The figure shows three views and two pictorial views of one solid part (mm, origin at its lowest corner). Answer the questions. A direction names the side the tool comes from. Give positions to 0.01 mm unless a question says otherwise; leave off trailing zeros. Order: outer loops, then holes, each group sorted by start corner. A loop starts at its lowest first (then second) coordinate and runs counter-clockwise, first axis right, second up. Notation, with made-up numbers: (-3, 22) - (42, 22) arc R16 cw to (42, 30) - close; hole circle Ø1 at (4, 43). An arc over 180 degrees is marked (long way). Answer as a JSON object with one key per item and string values. Group by question number.
Q1. The mould has two halves that part along X. Classify the marked faces 1, 2 and 3: released by +X, released by -X, zero draft, split by the parting line, or undercut.
Q2. Given pin 1 (4 mm diameter, centred on x = 20, y = 5, fed in from -Z); pin 2 (8 mm diameter, centred on x = 33.44, y = 10.56, fed in from -Z); pin 3 (4 mm diameter, centred on x = 26.5, z = 26.5, fed in from -Y); pin 4 (8 mm diameter, centred on x = 25.5, z = 9, fed in from -Y), each flat-ended and moving along its own axis, determine where each tip first touches the part or whether it passes through.
Q3. Consider line 1 (Y direction, x = 20, z = 23); line 2 (Z direction, x = 23, y = 45.5); line 3 (Y direction, x = 26, z = 31). Determine where each line is inside the solid, lowest interval first.
Q4. For the marked faces 4 and 5, determine the directions among +Z, -Z, +X, -X, +Y, -Y from which every point of the face is accessible in a straight line to the end or side of a thin tool.
Q5. A cutting plane is placed at B-B, the plane x = 20. Give the vertices of the cut face in (y, z), and give its area (3 significant figures).
Q6. A cutting plane is placed at C-C, the plane x = 33. Give the vertices of the cut face in (y, z), and give its area (3 significant figures).
Q7. A cutting plane is placed at D-D, the plane x = 15. Give the vertices of the cut face in (y, z) (3 decimals).
Q8. A cutting plane is placed at A-A, the plane y = 24. Give the vertices of the cut face in (x, z).
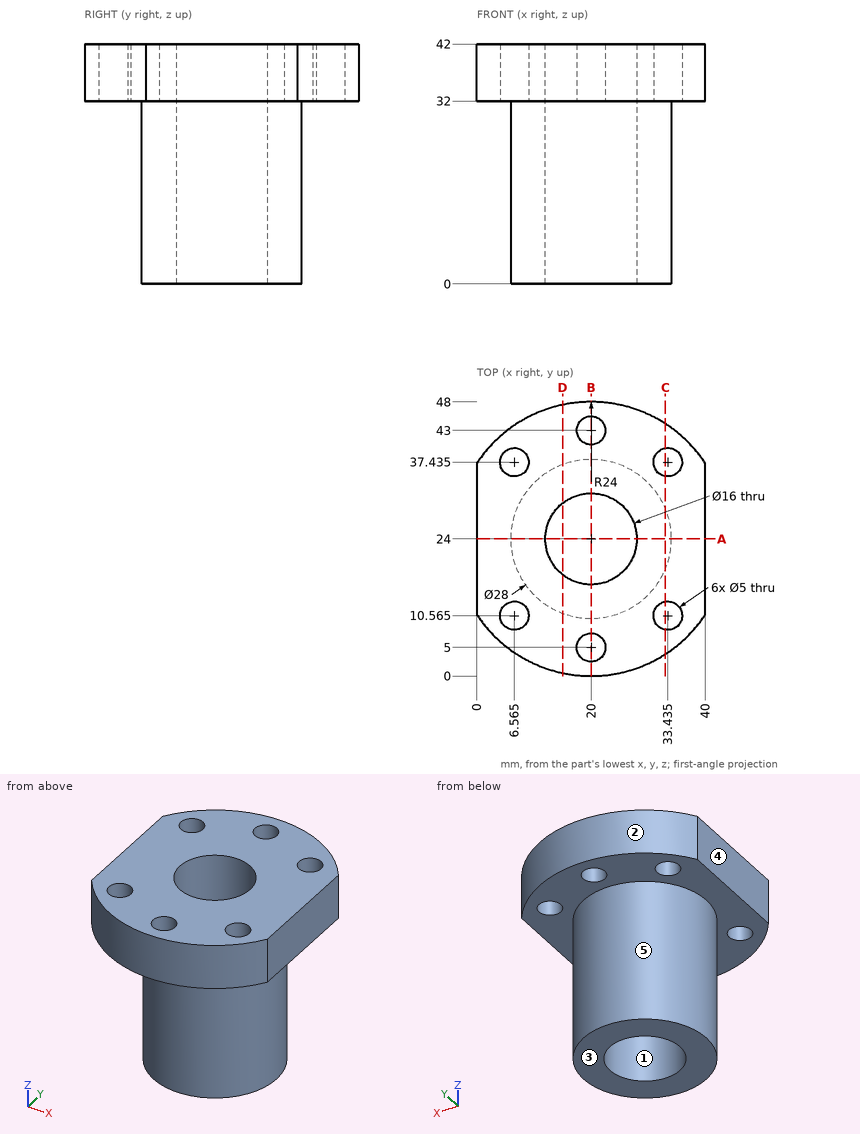
Reply:
{
 "1": {"face 1": "undercut", "face 2": "split by the parting line", "face 3": "zero draft"},
 "2": {"pin 1": "passes through", "pin 2": "stops at z = 32", "pin 3": "stops at y = 10.74", "pin 4": "stops at y = 10.08"},
 "3": {"line 1": "y = 10 to 16, 32 to 38", "line 2": "z = 32 to 42", "line 3": "y = 11.35 to 18.71, 29.29 to 36.65"},
 "4": {"face 4": "+Z, -Z, -X, +Y, -Y", "face 5": "-Z"},
 "5": {"outline": "(0, 32) - (2.5, 32) - (2.5, 42) - (0, 42) - close; (7.5, 32) - (10, 32) - (10, 0) - (16, 0) - (16, 42) - (7.5, 42) - close; (32, 0) - (38, 0) - (38, 32) - (40.5, 32) - (40.5, 42) - (32, 42) - close; (45.5, 32) - (48, 32) - (48, 42) - (45.5, 42) - close", "area": "604 mm^2"},
 "6": {"outline": "(3.83, 32) - (8.1, 32) - (8.1, 42) - (3.83, 42) - close; (13.03, 32) - (18.8, 32) - (18.8, 0) - (29.2, 0) - (29.2, 32) - (34.97, 32) - (34.97, 42) - (13.03, 42) - close; (39.9, 32) - (44.17, 32) - (44.17, 42) - (39.9, 42) - close", "area": "638 mm^2"},
 "7": {"outline": "(0.527, 32) - (10.923, 32) - (10.923, 0) - (17.755, 0) - (17.755, 42) - (0.527, 42) - close; (30.245, 0) - (37.077, 0) - (37.077, 32) - (47.473, 32) - (47.473, 42) - (30.245, 42) - close"},
 "8": {"outline": "(0, 32) - (6, 32) - (6, 0) - (12, 0) - (12, 42) - (0, 42) - close; (28, 0) - (34, 0) - (34, 32) - (40, 32) - (40, 42) - (28, 42) - close"}
}
